```python
from build123d import *

# Parameters (mm, degrees)
EXTRUDE_3_DEPTH     = 2
EXTRUDE_3_2_DEPTH   = 2
SKETCH_2_R          = 3.75
SKETCH_2_R_2        = 2.5
EXTRUDE_5_DEPTH     = 3
SKETCH_4_R          = 0.5
CUT_EXTRUDE_1_DEPTH = 2
SKETCH_5_R          = 2.5
EXTRUDE_7_DEPTH     = 1
SKETCH_1_2_R        = 3.75
EXTRUDE_1_DEPTH     = 2


with BuildPart() as part:
    # Sketch 1 → Extrude 3 (new body)
    with BuildSketch(Plane.XY):
        with BuildLine():
            Line((0, -2.497361401), (0.233236, -2.489096416))
            ThreePointArc((0.233236, -2.489096416), (2.5, 0), (0.233236, 2.489096416))
            Line((0.233236, 2.489096416), (0, 2.497361401))
            Line((0, 2.497361401), (-0.233236, 2.489096416))
            ThreePointArc((-0.233236, 2.489096416), (-2.5, 0), (-0.233236, -2.489096416))
            Line((-0.233236, -2.489096416), (0, -2.497361401))
        make_face()
    extrude(amount=EXTRUDE_3_DEPTH)



with BuildPart() as body_2:
    # Sketch 1 → Extrude 3 2 (new body)
    with BuildSketch(Plane.XY):
        with BuildLine():
            Line((14.07082784, 1.998745461), (2.88547071, 2.395111434))
            ThreePointArc((2.88547071, 2.395111434), (3.75, 0), (2.88547071, -2.395111434))
            Line((2.88547071, -2.395111434), (14.07082784, -1.998745461))
            ThreePointArc((14.07082784, -1.998745461), (16, 0), (14.07082784, 1.998745461))
        make_face()
    extrude(amount=EXTRUDE_3_2_DEPTH)

    # Sketch 4 → Cut-Extrude 1 (cut)
    with BuildSketch(Plane(origin=(0, 0, 0), x_dir=(-1, 0, 0), z_dir=(0, 0, -1))):
        with Locations((-14.5, 0)):
            Circle(SKETCH_4_R)
        with Locations((-4.5, 0)):
            Circle(SKETCH_4_R)
        with Locations((-6.5, 0)):
            Circle(SKETCH_4_R)
        with Locations((-8.5, 0)):
            Circle(SKETCH_4_R)
        with Locations((-10.5, 0)):
            Circle(SKETCH_4_R)
        with Locations((-12.5, 0)):
            Circle(SKETCH_4_R)
    extrude(amount=-CUT_EXTRUDE_1_DEPTH, mode=Mode.SUBTRACT)


with BuildPart() as body_3:
    # Sketch 2 → Extrude 5 (new body)
    with BuildSketch(Plane.XY.offset(2)):
        Circle(SKETCH_2_R)
        Circle(SKETCH_2_R_2, mode=Mode.SUBTRACT)
    extrude(amount=EXTRUDE_5_DEPTH)


with BuildPart() as body_4:
    # Sketch 5 → Extrude 7 (new body)
    with BuildSketch(Plane(origin=(0, 0, 0), x_dir=(-1, 0, 0), z_dir=(0, 0, -1))):
        Circle(SKETCH_5_R)
    extrude(amount=-EXTRUDE_7_DEPTH)


with BuildPart() as part_1:
    add(part.part)

    add(body_2.part)  # Extrude 1 merges body 2

    add(body_3.part)  # Extrude 1 merges body 3

    add(body_4.part)  # Extrude 1 merges body 4
    # Sketch 1 2 → Extrude 1 (add)
    with BuildSketch(Plane(origin=(0, 0, 2), x_dir=(-1, 0, 0), z_dir=(0, 0, -1))):
        with Locations(Location((0, 0, 0), (0, 0, 180))):
            Circle(SKETCH_1_2_R)
    extrude(amount=EXTRUDE_1_DEPTH)


solid = part_1.part
```
The listing builds one solid part. Answer for the finished solid, in the listing's coordinates (mm). A direction names the side the tool comes from. Coordinates: 2 decimals unless noted, no trailing zeros. Loops run counter-clockwise (first coordinate to the right, second up) from the corner with the lowest first, then second, coordinate; pieces in that order, holes last. Notation, with made-up numbers: M 52.25,4.25 L 111.25,4.25 A26 cw 111.25,34.25 Z; hole C 87,86.5 d4. An arc over 180 degrees is marked long. Answer as CSV lines item,"result". Start each with the question number.
(1) The part is cut by section D-D (y = -1). Give the vertices of the cut face in (x, z), and give its area (3 significant figures).
(2) For faces 1 (the flat face through (0, 0, 2)), 2 (the cylindrical face through (13, 0, 1)), determine the directions among +Z, -Z, +X, -X, +Y, -Y from which every point of the face is accessible in a straight line to the end or side of a thin tool.
(3) The part is cut by section C-C (x = 0). Give the vertices of the cut face in (y, z).
(4) The mould has two halves that part along Y. Classify faces 3 (the flat face through (3.8, -0.1, 0)), 4 (the cylindrical face through (-3.746, -0.165, 2.535)), 5 (the cylindrical face through (11, 0, 1)), 6 (the cylindrical face through (8, 0, 1)): pulls with the +Y half, pulls with the -Y half, needs draft (parallel to the pull), parting line crosses it, or undercut.
(5) The part is cut by section B-B (x = 10.5). Give the vertices of the cut face in (y, z).
(6) Find the intervals of material crossed by L1, parallel to Z at x = 10.25, y = -1; L2, parallel to Y at x = 14.5, z = 1.1; L3, parallel to Y at x = 8.5, z = 0.85, in increasing order. Write a range as [from, to].
(7) The part is cut by section A-A (z = 0.9). Give the vertices of the cut face in (x, y), and give its area (3 significant figures).
(8) Given pin 1 (1 mm diameter, centred on x = 5.5, y = -1, fed in from +Z); pin 2 (1 mm diameter, centred on y = -3, z = 1.5, fed in from -X); pin 3 (1 mm diameter, centred on x = 14, z = 2, fed in from +Y); pin 4 (2 mm diameter, centred on y = 0.5, z = 1, fed in from -X), each flat-ended and moving along its own axis, determine where each tip first touches the part or whether it passes through.
Determined:
1,outline,"M -3.61,0 L 15.73,0 L 15.73,2 L 3.61,2 L 3.61,5 L 2.29,5 L 2.29,2 L -2.29,2 L -2.29,5 L -3.61,5 Z"
1,area,"46.6 mm2"
2,face 1,"+Z"
2,face 2,"+Z, -Z"
3,outline,"M -3.75,0 L 3.75,0 L 3.75,5 L 2.5,5 L 2.5,2 L -2.5,2 L -2.5,5 L -3.75,5 Z"
4,face 3,"needs draft"
4,face 4,"parting line crosses it"
4,face 5,"undercut"
4,face 6,"undercut"
5,outline,"M -2.13,0 L -0.5,0 L -0.5,2 L -2.13,2 Z; M 0.5,0 L 2.13,0 L 2.13,2 L 0.5,2 Z"
6,L1,"[0, 2]"
6,L2,"[-1.94, -0.5], [0.5, 1.94]"
6,L3,"[-2.2, -0.5], [0.5, 2.2]"
7,outline,"M 2.89,-2.4 L 14.07,-2 A2 ccw 14.07,2 L 2.89,2.4 A3.75 ccw long Z; hole C 4.5,0 d1; hole C 6.5,0 d1; hole C 8.5,0 d1; hole C 10.5,0 d1; hole C 12.5,0 d1; hole C 14.5,0 d1"
7,area,"91.8 mm2"
8,pin 1,"z = 2"
8,pin 2,"x = -2.8"
8,pin 3,"y = 2.02"
8,pin 4,"x = -3.75"
